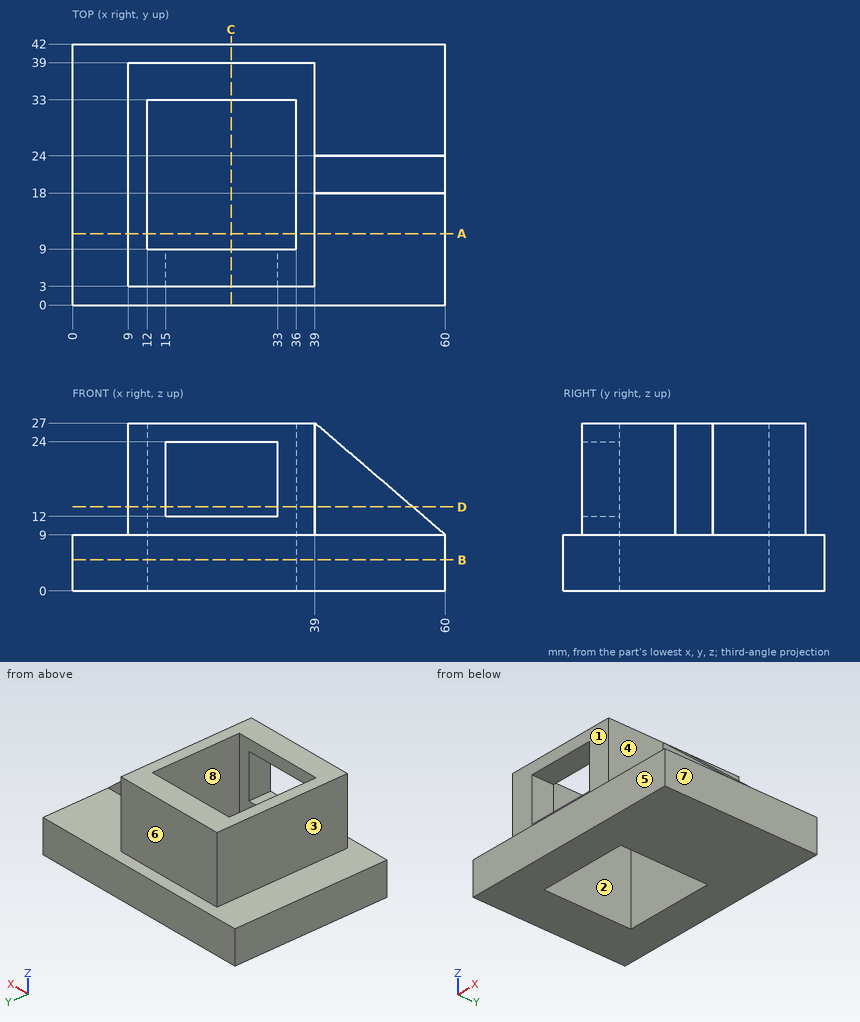
Input: dimensioned drawing with shaded views. Units: mm. Origin: part minimum x, y, z. A direction names the side the tool comes from. Give positions to 0.01 mm unless a question says otherwise; leave off trailing zeros. Loops run counter-clockwise (first coordinate to the right, second up) from the corner with the lowest first, then second, coordinate; pieces in that order, holes last. Notation, with made-up numbers: (16, 87) - (34, 87) arc R19 ccw to (34, 115) - close; hole circle Ø5 at (28.25, 29). An arc over 180 degrees is marked (long way). Answer as CSV lines item,"result". Start each with the question number.
(1) Mould query, pull axis Y, two halves, no side actions, for the marked faces 5, 6, 7 and 8. Classes: +Y half, -Y half, draft (parallel to the pull), parting line (faces both ways), or undercut.
(2) Section query D-D (z = 13.5). Output: boundary loops of the cut face in (x, y).
(3) Section query A-A (y = 11.5). Output: boundary loops of the cut face in (x, z).
(4) Reachability of the marked faces 1, 2, 3 and 4 from +Z, -Z, +X, -X, +Y, -Y: full face, straight path, thin tool, end or side. Return the list, or none.
(5) Section query B-B (z = 5). Output: boundary loops of the cut face in (x, y).
(6) Pin query (flat end, axial travel): P1, Ø14.5, axis at x = 46.5, z = 19, coming from the +Y side; P2, Ø7, axis at x = 29, z = 17, coming from the +Y side; P3, Ø4.5, axis at y = 30.5, z = 18, coming from the +X side; P4, Ø5, axis at x = 33, y = 26.5, coming from the +Z side (3 decimals). Return the tip coordinate at first contact, or that it passes through.
(7) Ray query, line 1 along X through (y, z) = (29.5, 25.75); line 2 along X through (y, z) = (4.5, 23.25); line 3 along Y through (x, z) = (29, 3). Return the intervals inside material, ascending. Write a range as [from, to].
(8) Section query C-C (x = 25.5). Output: boundary loops of the cut face in (y, z).
Worked answers:
1,face 5,"-Y half"
1,face 6,"+Y half"
1,face 7,"draft"
1,face 8,"undercut"
2,outline,"(9, 3) - (15, 3) - (15, 9) - (12, 9) - (12, 33) - (36, 33) - (36, 9) - (33, 9) - (33, 3) - (39, 3) - (39, 18) - (54.75, 18) - (54.75, 24) - (39, 24) - (39, 39) - (9, 39) - close"
3,outline,"(0, 0) - (12, 0) - (12, 27) - (9, 27) - (9, 9) - (0, 9) - close; (36, 0) - (60, 0) - (60, 9) - (39, 9) - (39, 27) - (36, 27) - close"
4,face 1,"+Z, +X, -X, -Y"
4,face 2,"+Z, -Z"
4,face 3,"+Z, -X, +Y, -Y"
4,face 4,"+Z, +X, -Y"
5,outline,"(0, 0) - (60, 0) - (60, 42) - (0, 42) - close; hole (12, 9) - (36, 9) - (36, 33) - (12, 33) - close"
6,P1,"stops at y = 24"
6,P2,"stops at y = 39"
6,P3,"stops at x = 39"
6,P4,"passes through"
7,line 1,"x = [9, 12], [36, 39]"
7,line 2,"x = [9, 15], [33, 39]"
7,line 3,"y = [0, 9], [33, 42]"
8,outline,"(0, 0) - (9, 0) - (9, 12) - (3, 12) - (3, 9) - (0, 9) - close; (3, 24) - (9, 24) - (9, 27) - (3, 27) - close; (33, 0) - (42, 0) - (42, 9) - (39, 9) - (39, 27) - (33, 27) - close"
